Part print with two shaded views. Sizes in mm from the minimum x, y, z corner. A direction names the side the tool comes from. Round coordinates to 2 decimals unless told otherwise and drop trailing zeros. Write each loop counter-clockwise with the first axis right and the second up, starting at its lowest first coordinate (ties: lowest second). Pieces come first, ordered by that corner, then holes.
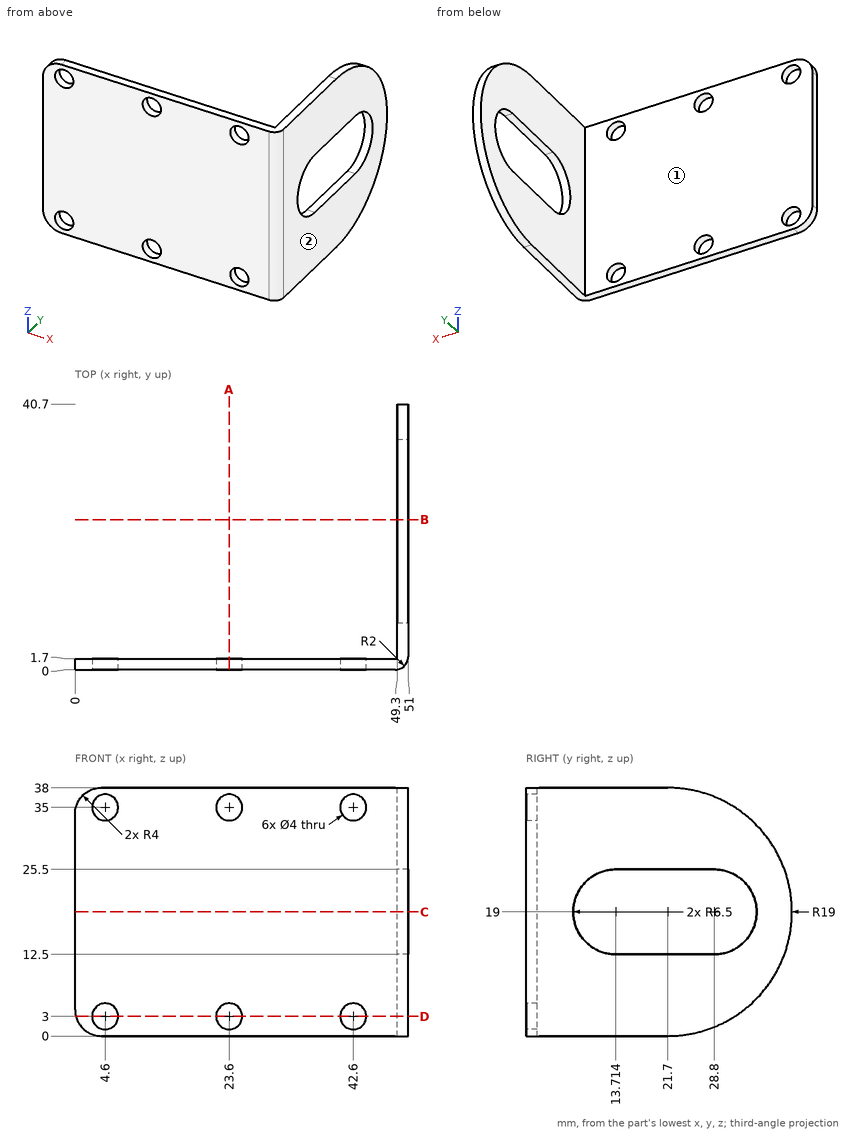
Q1. Cut at B-B on y = 23. Write the cut outline in (x, z).
Values follow:
outline: (49.3, 0.04) - (51, 0.04) - (51, 12.5) - (49.3, 12.5) - close; (49.3, 25.5) - (51, 25.5) - (51, 37.96) - (49.3, 37.96) - close
Q2. Which spindle directions (+Z, -Z, +X, -X, +Y, -Y) get a long thin tool onto all of the face, cutting with end or side? Do the marked faces 1 and 2. Say none if no direction does.
Values follow:
face 1: +Z, -Z, -X, +Y
face 2: +Z, -Z, +X, +Y, -Y
Q3. Drop flat-ended pins along their axis: pin 1 (4.5 mm diameter, centred on x = 42.6, z = 35, fed in from +Y); pin 2 (6 mm diameter, centred on y = 14.5, z = 5, fed in from -X). Give the stop position or say it passes through.
Values follow:
pin 1: stops at y = 1.7
pin 2: stops at x = 49.3
Q4. Wall check: L1, parallel to X at y = 1.2, z = 35; L2, parallel to X at y = 5, z = 11.5; L3, parallel to Y at x = 31, z = 34. Give the ranges that are in metal, low to high.
Values follow:
L1: x = 0.13 to 2.6, 6.6 to 21.6, 25.6 to 40.6, 44.6 to 50.83
L2: x = 49.3 to 51
L3: y = 0 to 1.7
Q5. Cut at A-A on x = 23.6. Write the cut outline in (y, z), plus the area to 3 significant figures.
Values follow:
outline: (0, 0) - (1.7, 0) - (1.7, 1) - (0, 1) - close; (0, 5) - (1.7, 5) - (1.7, 33) - (0, 33) - close; (0, 37) - (1.7, 37) - (1.7, 38) - (0, 38) - close
area: 51.0 mm2
Q6. Cut at D-D on z = 3. Write the cut outline in (x, y).
Values follow:
outline: (0.13, 0) - (2.6, 0) - (2.6, 1.7) - (0.13, 1.7) - close; (6.6, 0) - (21.6, 0) - (21.6, 1.7) - (6.6, 1.7) - close; (25.6, 0) - (40.6, 0) - (40.6, 1.7) - (25.6, 1.7) - close; (44.6, 0) - (49, 0) arc R2 ccw to (51, 2) - (51, 31.95) - (49.3, 31.95) - (49.3, 1.7) - (44.6, 1.7) - close
Q7. Cut at C-C on z = 19. Write the cut outline in (x, y), plus the area to 3 significant figures.
Values follow:
outline: (0, 0) - (49, 0) arc R2 ccw to (51, 2) - (51, 7.21) - (49.3, 7.21) - (49.3, 1.7) - (0, 1.7) - close; (49.3, 35.3) - (51, 35.3) - (51, 40.7) - (49.3, 40.7) - close
area: 104 mm2
